Check sheet for the modelled part. Datum: model origin and axes. Units: mm. Face numbers are marked on the shaded views. A direction names the side the tool comes from. Coordinates: 2 decimals unless noted, no trailing zeros. Loops run counter-clockwise (first coordinate to the right, second up) from the corner with the lowest first, then second, coordinate; pieces in that order, holes last. Notation, with made-up numbers: (-22.75, 4) - (6.25, 4) arc R9 ccw to (6.25, 9) - close; hole circle Ø9 at (-31.5, -27). An arc over 180 degrees is marked (long way). Write each question's results on one line, items separated by ' | '. Start each with the question number.
1. Thickness scan on line 1 (X direction, y = 60, z = 12); line 2 (X direction, y = 3, z = 1); line 3 (Y direction, x = -6.5, z = 19). Record the ranges inside material, lowest first. Write a range as [from, to].
2. Draft check along Y on the marked faces 1, 2 and 3. Enter one of: released by +Y, released by -Y, zero draft, split by the parting line, or undercut.
3. Cross-section at B-B (z = -21). Record the cut outline in (x, y), and give its area (3 significant figures).
4. Tool access check on the marked faces 4, 5, 6 and 7. Record the directions out of +Z, -Z, +X, -X, +Y, -Y that give a thin tool (end or side, any length) a straight path to the whole face; none if there is none.
5. Cross-section at C-C (y = 92). Record the cut outline in (x, z).
6. Gauge pin test, flat ends, axial feed: P1, Ø1.4, axis at x = 0, z = 62.5, coming from the -Y side; P2, Ø1.5, axis at x = -8, y = 68, coming from the -Z side; P3, Ø4, axis at y = 40.5, z = 26.5, coming from the -X side; P4, Ø3, axis at y = 19, z = -21, coming from the -X side. Record the tip position at first contact, or that the pin passes through.
7. Cross-section at A-A (y = 19). Record the cut outline in (x, z).
```python
from build123d import *

# Parameters (mm, degrees)
SKETCH_1_W             = 67
SKETCH_1_H             = 62
EXTRUDE_1_DEPTH        = 10
SKETCH_3_W             = 14
SKETCH_3_H             = 20
EXTRUDE_2_DEPTH        = 12.5
SKETCH_4_W             = 10
SKETCH_4_H             = 65
EXTRUDE_3_DEPTH        = 67
SKETCH_5_W             = 67
SKETCH_5_H             = 44
EXTRUDE_4_DEPTH        = 8
EXTRUDE_5_DEPTH        = 20
CUT_EXTRUDE_START      = -6
CUT_EXTRUDE_1_DEPTH    = 8
EXTRUDE_6_DEPTH        = 6
SKETCH_9_R             = 3
CUT_EXTRUDE_2_DEPTH    = 23
SKETCH_10_W            = 24
SKETCH_10_H            = 23.8
EXTRUDE_7_DEPTH        = 8
SKETCH_12_W            = 14
SKETCH_12_H            = 20
EXTRUDE_8_DEPTH        = 11.5
SKETCH_13_R            = 0.95
CUT_EXTRUDE_4_DEPTH    = 8
SKETCH_14_W            = 7.5
SKETCH_14_H            = 6
SKETCH_14_W_2          = 8
EXTRUDE_9_DEPTH        = 11.8
SKETCH_15_R            = 0.95
CUT_EXTRUDE_5_DEPTH    = 11.8
SKETCH_16_W            = 3
SKETCH_16_H            = 6
EXTRUDE_10_DEPTH       = 12
FILLET_1_RADIUS        = 3
FILLET_1_LENGTH        = 3
SKETCH_17_R            = 1.75
CUT_EXTRUDE_6_DEPTH    = 7
SKETCH_18_R            = 5
EXTRUDE_11_DEPTH       = 45
FILLET_2_R             = 3
FILLET_2_OF_MIRROR_1_R = 3
SKETCH_20_R            = 1.75
CUT_EXTRUDE_7_DEPTH    = 35
SKETCH_21_W            = 15
SKETCH_21_H            = 55
CUT_EXTRUDE_8_DEPTH    = 35
SKETCH_24_R            = 1.75
CUT_EXTRUDE_11_DEPTH   = 18
SKETCH_25_R            = 1.5
CUT_EXTRUDE_12_DEPTH   = 10
FILLET_3_R             = 4
EXTRUDE_12_DEPTH       = 3
SKETCH_27_W            = 9.9
SKETCH_27_H            = 3.8
EXTRUDE_13_DEPTH       = 1
SKETCH_29_R            = 1.4
CUT_EXTRUDE_13_DEPTH   = 4


with BuildPart() as part:
    # 草图1 → 凸台-拉伸1 (new body)
    with BuildSketch(Plane(origin=(0, 0, 0), x_dir=(1, 0, 0), z_dir=(0, 1, 0))):
        Rectangle(SKETCH_1_W, SKETCH_1_H)
    extrude(amount=EXTRUDE_1_DEPTH)

    # 草图3 → 凸台-拉伸2 (add)
    with BuildSketch(Plane(origin=(0, 10, 0), x_dir=(1, 0, 0), z_dir=(0, 1, 0))):
        with Locations((-26.5, 26)):
            Rectangle(SKETCH_3_W, SKETCH_3_H)
    extrude(amount=EXTRUDE_2_DEPTH)

    # 草图4 → 凸台-拉伸3 (add)
    with BuildSketch(Plane.ZY.offset(33.5)):
        with Locations((-11, 42.5)):
            Rectangle(SKETCH_4_W, SKETCH_4_H)
    extrude(amount=-EXTRUDE_3_DEPTH)

    # 草图5 → 凸台-拉伸4 (add)
    with BuildSketch(Plane(origin=(0, 75, 0), x_dir=(1, 0, 0), z_dir=(0, 1, 0))):
        with Locations((0, -6)):
            Rectangle(SKETCH_5_W, SKETCH_5_H)
    extrude(amount=-EXTRUDE_4_DEPTH)

    # 草图6 → 凸台-拉伸5 (add)
    with BuildSketch(Plane(origin=(33.5, 0, 0), x_dir=(0, 0, -1), z_dir=(1, 0, 0))):
        with BuildLine():
            Line((-28, 60), (-28, 67))
            Line((-28, 67), (-8, 67))
            Line((-8, 67), (-8, 60))
            ThreePointArc((-8, 60), (-18, 50), (-28, 60))
        make_face()
    extrude_5 = extrude(amount=-EXTRUDE_5_DEPTH)

    # 草图7 → 切除-拉伸1 (cut)
    with BuildSketch(Plane(origin=(33.5, 0, 0), x_dir=(0, 0, -1), z_dir=(1, 0, 0)).offset(CUT_EXTRUDE_START)):
        with BuildLine():
            Line((-28, 60), (-28, 70.000230089))
            Line((-28, 70.000230089), (-8, 70.000230089))
            Line((-8, 70.000230089), (-8, 60))
            ThreePointArc((-8, 60), (-18, 50), (-28, 60))
        make_face()
    cut_extrude_1 = extrude(amount=-CUT_EXTRUDE_1_DEPTH, mode=Mode.SUBTRACT)

    # 草图8 → 凸台-拉伸6 (add)
    with BuildSketch(Plane(origin=(0, 75, 0), x_dir=(1, 0, 0), z_dir=(0, 1, 0))):
        Polygon((0, -68), (10, -68), (23.694211345, -28), (0, -28), align=None)
    extrude_6 = extrude(amount=-EXTRUDE_6_DEPTH)

    # 草图9 → 切除-拉伸2 (cut)
    with BuildSketch(Plane(origin=(33.5, 0, 0), x_dir=(0, 0, -1), z_dir=(1, 0, 0))):
        with Locations((-18, 60)):
            Circle(SKETCH_9_R)
    cut_extrude_2 = extrude(amount=-CUT_EXTRUDE_2_DEPTH, mode=Mode.SUBTRACT)

    # 草图10 → 凸台-拉伸7 (add)
    with BuildSketch(Plane(origin=(29.7887098, 0, 10.198322192), x_dir=(0.32389942978753467, 0, -0.9460915174460186), z_dir=(0.9460915174460186, 0, 0.32389942978753467))):
        Polygon((-44, 75), (-15, 75), (-15, 40.2), (-43, 40.2), (-49, 40.2), (-49, 75), align=None)
        with Locations((-32, 57.1)):
            Rectangle(SKETCH_10_W, SKETCH_10_H, mode=Mode.SUBTRACT)
    extrude_7 = extrude(amount=-EXTRUDE_7_DEPTH)

    # 草图12 → 凸台-拉伸8 (add)
    with BuildSketch(Plane(origin=(0, 75, 0), x_dir=(1, 0, 0), z_dir=(0, 1, 0))):
        with Locations((-26.5, 26)):
            Rectangle(SKETCH_12_W, SKETCH_12_H)
    extrude(amount=-EXTRUDE_8_DEPTH)

    # 草图13 → 切除-拉伸4 (cut)
    with BuildSketch(Plane(origin=(22.21997766, 0, 7.607126754), x_dir=(-0.3238994297875346, 0, 0.9460915174460185), z_dir=(-0.9460915174460185, 0, -0.3238994297875346))):
        with Locations((38.5, 70.95)):
            Circle(SKETCH_13_R)
        with Locations((26.5, 70.95)):
            Circle(SKETCH_13_R)
        with Locations((26.5, 43.25)):
            Circle(SKETCH_13_R)
        with Locations((38.5, 43.25)):
            Circle(SKETCH_13_R)
    cut_extrude_4 = extrude(amount=-CUT_EXTRUDE_4_DEPTH, mode=Mode.SUBTRACT)

    # 草图14 → 凸台-拉伸9 (add)
    with BuildSketch(Plane(origin=(0, 75, 0), x_dir=(1, 0, 0), z_dir=(0, 1, 0))):
        with Locations((7.95, -5)):
            Rectangle(SKETCH_14_W, SKETCH_14_H)
        with Locations((8.2, -34.8)):
            Rectangle(SKETCH_14_W_2, SKETCH_14_H)
    extrude(amount=EXTRUDE_9_DEPTH)

    # 草图15 → 切除-拉伸5 (cut)
    with BuildSketch(Plane.ZY.offset(-4.2)):
        with Locations((33.75, 81.5)):
            Circle(SKETCH_15_R)
        with Locations((6.05, 81.5)):
            Circle(SKETCH_15_R)
    extrude(amount=-CUT_EXTRUDE_5_DEPTH, mode=Mode.SUBTRACT)

    # 草图16 → 凸台-拉伸10 (add)
    with BuildSketch(Plane(origin=(0, 75, 0), x_dir=(1, 0, 0), z_dir=(0, 1, 0))):
        with Locations((0, -63)):
            Rectangle(SKETCH_16_W, SKETCH_16_H)
    extrude(amount=EXTRUDE_10_DEPTH)

    # 圆角1: full round fillet: the end face becomes a half cylinder, R = half its width
    fillet_1_face = Plane((0, 87, 63), x_dir=(1, 0, 0), z_dir=(0, 1, 0))  # on the end face: x along it, z out of the body
    fillet_1_slab = fillet_1_face.offset(-FILLET_1_RADIUS / 2) * Box(FILLET_1_LENGTH, 2 * FILLET_1_RADIUS, FILLET_1_RADIUS, mode=Mode.PRIVATE)  # the body's end, R deep
    fillet_1_round = Plane((0, 84, 63), x_dir=(0, 1, 0), z_dir=(1, 0, 0)) * Cylinder(FILLET_1_RADIUS, FILLET_1_LENGTH, mode=Mode.PRIVATE)  # its axis R under the face
    add(fillet_1_slab - fillet_1_round, mode=Mode.SUBTRACT)

    # 草图17 → 切除-拉伸6 (cut)
    with BuildSketch(Plane.ZY.offset(1.5)):
        with Locations((63, 84)):
            Circle(SKETCH_17_R)
    extrude(amount=-CUT_EXTRUDE_6_DEPTH, mode=Mode.SUBTRACT)

    # 草图18 → 凸台-拉伸11 (add)
    with BuildSketch(Plane(origin=(0, 75, 0), x_dir=(1, 0, 0), z_dir=(0, 1, 0))):
        with Locations(Location((10, 6, 0), (0, 0, 90))):
            Circle(SKETCH_18_R)
    extrude_11 = extrude(amount=EXTRUDE_11_DEPTH)

    # 圆角2
    fillet_2_edges = [part.edges().sort_by_distance(p)[0] for p in [
        (10, 75, -1),
    ]]
    fillet(fillet_2_edges, radius=FILLET_2_R - 0.0001)  # a hair under: the kernel refuses the full size

    # 镜向1: 凸台-拉伸5, 切除-拉伸1, 凸台-拉伸6, 切除-拉伸2, 凸台-拉伸7, 切除-拉伸4, 凸台-拉伸11 across plane
    add(extrude_5.mirror(Plane(origin=(0, 0, 0), x_dir=(0, 0, 1), z_dir=(1, 0, 0))))
    add(cut_extrude_1.mirror(Plane(origin=(0, 0, 0), x_dir=(0, 0, 1), z_dir=(1, 0, 0))), mode=Mode.SUBTRACT)
    add(extrude_6.mirror(Plane(origin=(0, 0, 0), x_dir=(0, 0, 1), z_dir=(1, 0, 0))))
    add(cut_extrude_2.mirror(Plane(origin=(0, 0, 0), x_dir=(0, 0, 1), z_dir=(1, 0, 0))), mode=Mode.SUBTRACT)
    add(extrude_7.mirror(Plane(origin=(0, 0, 0), x_dir=(0, 0, 1), z_dir=(1, 0, 0))))
    add(cut_extrude_4.mirror(Plane(origin=(0, 0, 0), x_dir=(0, 0, 1), z_dir=(1, 0, 0))), mode=Mode.SUBTRACT)
    add(extrude_11.mirror(Plane(origin=(0, 0, 0), x_dir=(0, 0, 1), z_dir=(1, 0, 0))))

    # 圆角2 of 镜向1
    fillet_2_of_mirror_1_edges = [part.edges().sort_by_distance(p)[0] for p in [
        (-10, 75, -1),
    ]]
    fillet(fillet_2_of_mirror_1_edges, radius=FILLET_2_OF_MIRROR_1_R - 0.0001)  # a hair under: the kernel refuses the full size

    # 草图20 → 切除-拉伸7 (cut)
    with BuildSketch(Plane.ZY.offset(33.5)):
        with Locations((-31, 67)):
            Circle(SKETCH_20_R)
        with Locations((-21, 67)):
            Circle(SKETCH_20_R)
        with Locations((-31, 19)):
            Circle(SKETCH_20_R)
        with Locations((-21, 19)):
            Circle(SKETCH_20_R)
    extrude(amount=-CUT_EXTRUDE_7_DEPTH, mode=Mode.SUBTRACT)

    # 草图21 → 切除-拉伸8 (cut)
    with BuildSketch(Plane(origin=(0, 0, -16), x_dir=(-1, 0, 0), z_dir=(0, 0, -1))):
        with Locations((0, 37.5)):
            Rectangle(SKETCH_21_W, SKETCH_21_H)
    extrude(amount=-CUT_EXTRUDE_8_DEPTH, mode=Mode.SUBTRACT)

    # 草图24 → 切除-拉伸11 (cut)
    with BuildSketch(Plane(origin=(0, 10, 0), x_dir=(1, 0, 0), z_dir=(0, 1, 0))):
        with Locations(Location((-10, -21, 0), (0, 0, 270))):
            Circle(SKETCH_24_R)
        with Locations(Location((10, -21, 0), (0, 0, 270))):
            Circle(SKETCH_24_R)
        with Locations(Location((-10, -1, 0), (0, 0, 270))):
            Circle(SKETCH_24_R)
        with Locations(Location((10, -1, 0), (0, 0, 270))):
            Circle(SKETCH_24_R)
    extrude(amount=-CUT_EXTRUDE_11_DEPTH, mode=Mode.SUBTRACT)

    # 草图25 → 切除-拉伸12 (cut)
    with BuildSketch(Plane(origin=(0, 120, 0), x_dir=(1, 0, 0), z_dir=(0, 1, 0))):
        with Locations(Location((10, 6, 0), (0, 0, 270))):
            Circle(SKETCH_25_R)
        with Locations(Location((-10, 6, 0), (0, 0, 270))):
            Circle(SKETCH_25_R)
    extrude(amount=-CUT_EXTRUDE_12_DEPTH, mode=Mode.SUBTRACT)

    # 圆角3
    fillet_3_edges = [part.edges().sort_by_distance(p)[0] for p in [
        (-1.5, 75, 63),
        (1.5, 75, 63),
    ]]
    fillet(fillet_3_edges, radius=FILLET_3_R)

    # 草图26 → 凸台-拉伸12 (add)
    with BuildSketch(Plane.XZ.offset(-69)):
        Polygon((-6.348905601, 53.965611109), (6.348905601, 53.965611109), (13.91763774, 56.556806547), (10, 68), (-10, 68), (-13.91763774, 56.556806547), align=None)
    extrude(amount=EXTRUDE_12_DEPTH)

    # 草图27 → 凸台-拉伸13 (add)
    with BuildSketch(Plane.XZ.offset(-66)):
        with Locations((0, 62)):
            Rectangle(SKETCH_27_W, SKETCH_27_H)
    extrude(amount=EXTRUDE_13_DEPTH)

    # 草图29 → 切除-拉伸13 (cut)
    with BuildSketch(Plane.XZ.offset(-65)):
        with Locations(Location((0, 62, 0), (0, 0, 270))):
            Circle(SKETCH_29_R)
    extrude(amount=-CUT_EXTRUDE_13_DEPTH, mode=Mode.SUBTRACT)


solid = part.part
```
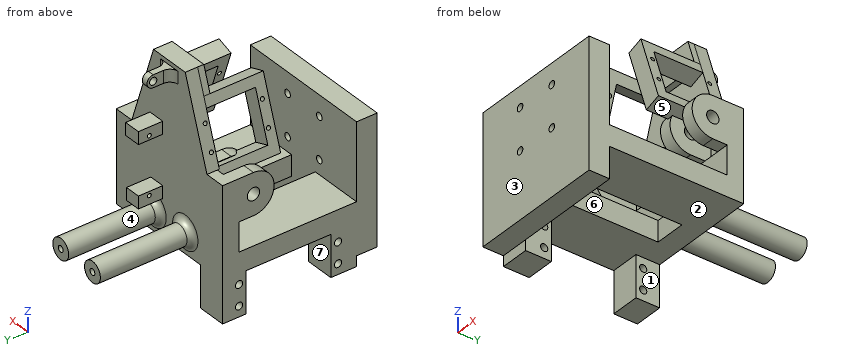
Established:
1) line 1: [-33.5, -27.5], [-19.5, -13.5], [13.5, 19.5], [27.5, 33.5] | line 2: [-33.5, -11.75], [-8.25, 8.25], [11.75, 33.5] | line 3: [0, 10], [67, 75]
2) face 1: zero draft | face 2: undercut | face 3: released by -Y
3) outline: (-33.5, 0) - (33.5, 0) - (33.5, 10) - (-19.5, 10) - (-19.5, 17.25) - (-33.5, 17.25) - close; (-33.5, 20.75) - (-19.5, 20.75) - (-19.5, 22.5) - (-33.5, 22.5) - close; (-33.5, 63.5) - (-19.5, 63.5) - (-19.5, 65.25) - (-33.5, 65.25) - close; (-33.5, 68.75) - (-19.5, 68.75) - (-19.5, 75) - (-33.5, 75) - close | area: 908 mm^2
4) face 4: +Y | face 5: none | face 6: -Z | face 7: -Z, +X, -X
5) outline: circle Ø10 at (-10, -6); circle Ø10 at (10, -6)
6) P1: y = 69 | P2: z = -16 | P3: x = -24.89 | P4: through
7) outline: (-33.5, -36) - (-19.5, -36) - (-19.5, -32.75) - (-33.5, -32.75) - close; (-33.5, -29.25) - (-19.5, -29.25) - (-19.5, -22.75) - (-33.5, -22.75) - close; (-33.5, -19.25) - (-19.5, -19.25) - (-19.5, -16) - (-7.5, -16) - (-7.5, -6) - (-33.5, -6) - close; (7.5, -16) - (33.5, -16) - (33.5, -6) - (7.5, -6) - close
